Geometry check sheet. Reference: the model listing, model coordinates, mm. A direction names the side the tool comes from. Round coordinates to 2 decimals unless told otherwise and drop trailing zeros. Loops run counter-clockwise (first coordinate to the right, second up) from the corner with the lowest first, then second, coordinate; pieces in that order, holes last. Notation, with made-up numbers: (81, -18) - (124, -18) arc R16 ccw to (124, -14) - close; hole circle Ø2 at (-37, 59). An arc over 180 degrees is marked (long way). Answer as CSV lines item,"result". Start each with the question number.
1) Draft check along X on faces 3 (the cylindrical face through (98.013, 3.131, -136.616)), 4 (the flat face through (79, 0, -132)), 5 (the flat face through (160, 3, -128)). Enter one of: released by +X, released by -X, zero draft, split by the parting line, or undercut.
2) Depth check by flat-ended pin: P1, Ø3.5, axis at x = 118.12, z = -223.04, coming from the +Y side. Enter the tip coordinate at first touch or a pass-through.
3) Access from +Z, -Z, +X, -X, +Y, -Y to the whole of each face (thin tool, end or side, straight path). Record for faces 1 (the flat face through (71.65, 3, -10)), 2 (the flat face through (79, 3, -260)).
4) Cross-section at A-A on z = -45. Record the boundary of the cut face in (x, y), and give its area (4 significant figures).
5) Cross-section at C-C on y = 4.75. State how many separate pieces and enclosed holes the cut face has, and give its area (3 significant figures).
6) Cross-section at B-B on z = -193. Record the boundary of the cut face in (x, y).
7) Thickness scan on line 1 along X through (y, z) = (4.5, -170); line 2 along X through (y, z) = (4, -169.5); line 3 along Z through (x, y) = (84, 0.75). Record the ranges inside material, lowest first.
from build123d import *

# Parameters (mm, degrees)
SKETCH1_W           = 160
SKETCH1_H           = 260
SKETCH1_R           = 35
SKETCH1_R_2         = 25
SKETCH1_R_3         = 2.25
SKETCH1_R_4         = 1.175
SKETCH1_R_5         = 1.65
BOSS_EXTRUDE1_DEPTH = 6.35


with BuildPart() as part:
    # Sketch1 → Boss-Extrude1 (new body)
    with BuildSketch(Plane(origin=(0, 0, 0), x_dir=(1, 0, 0), z_dir=(0, 1, 0))):
        with Locations((80, 130)):
            Rectangle(SKETCH1_W, SKETCH1_H)
        with Locations(Location((87.5, 170, 0), (0, 0, 270))):
            Circle(SKETCH1_R, mode=Mode.SUBTRACT)
        with Locations(Location((87.5, 45, 0), (0, 0, 270))):
            Circle(SKETCH1_R_2, mode=Mode.SUBTRACT)
        with Locations(Location((148.75, 170, 0), (0, 0, 270))):
            Circle(SKETCH1_R_3, mode=Mode.SUBTRACT)
        with Locations(Location((118.125, 116.955944018, 0), (0, 0, 270))):
            Circle(SKETCH1_R_3, mode=Mode.SUBTRACT)
        with Locations(Location((56.875, 116.955944018, 0), (0, 0, 270))):
            Circle(SKETCH1_R_3, mode=Mode.SUBTRACT)
        with Locations(Location((26.25, 170, 0), (0, 0, 270))):
            Circle(SKETCH1_R_3, mode=Mode.SUBTRACT)
        with Locations(Location((56.875, 223.044055982, 0), (0, 0, 270))):
            Circle(SKETCH1_R_3, mode=Mode.SUBTRACT)
        with Locations(Location((118.125, 223.044055982, 0), (0, 0, 270))):
            Circle(SKETCH1_R_3, mode=Mode.SUBTRACT)
        with Locations(Location((5.475532842, 135.298909731, 0), (0, 0, 270))):
            Circle(SKETCH1_R_4, mode=Mode.SUBTRACT)
        with Locations(Location((9.516263037, 126.701090269, 0), (0, 0, 270))):
            Circle(SKETCH1_R_4, mode=Mode.SUBTRACT)
        with Locations(Location((10, 250, 0), (0, 0, 270))):
            Circle(SKETCH1_R_5, mode=Mode.SUBTRACT)
        with Locations(Location((30, 250, 0), (0, 0, 270))):
            Circle(SKETCH1_R_5, mode=Mode.SUBTRACT)
        with Locations(Location((50, 250, 0), (0, 0, 270))):
            Circle(SKETCH1_R_5, mode=Mode.SUBTRACT)
        with Locations(Location((70, 250, 0), (0, 0, 270))):
            Circle(SKETCH1_R_5, mode=Mode.SUBTRACT)
        with Locations(Location((90, 250, 0), (0, 0, 270))):
            Circle(SKETCH1_R_5, mode=Mode.SUBTRACT)
        with Locations(Location((110, 250, 0), (0, 0, 270))):
            Circle(SKETCH1_R_5, mode=Mode.SUBTRACT)
        with Locations(Location((130, 250, 0), (0, 0, 270))):
            Circle(SKETCH1_R_5, mode=Mode.SUBTRACT)
        with Locations(Location((150, 250, 0), (0, 0, 270))):
            Circle(SKETCH1_R_5, mode=Mode.SUBTRACT)
        with BuildLine():
            Line((8.35, 6.5), (8.35, 13.5))
            ThreePointArc((8.35, 13.5), (10, 15.15), (11.65, 13.5))
            Line((11.65, 13.5), (11.65, 6.5))
            ThreePointArc((11.65, 6.5), (10, 4.85), (8.35, 6.5))
        make_face(mode=Mode.SUBTRACT)
        with BuildLine():
            Line((31.65, 6.5), (31.65, 13.5))
            ThreePointArc((31.65, 13.5), (30, 15.15), (28.35, 13.5))
            Line((28.35, 13.5), (28.35, 6.5))
            ThreePointArc((28.35, 6.5), (30, 4.85), (31.65, 6.5))
        make_face(mode=Mode.SUBTRACT)
        with BuildLine():
            Line((51.65, 6.5), (51.65, 13.5))
            ThreePointArc((51.65, 13.5), (50, 15.15), (48.35, 13.5))
            Line((48.35, 13.5), (48.35, 6.5))
            ThreePointArc((48.35, 6.5), (50, 4.85), (51.65, 6.5))
        make_face(mode=Mode.SUBTRACT)
        with BuildLine():
            Line((71.65, 6.5), (71.65, 13.5))
            ThreePointArc((71.65, 13.5), (70, 15.15), (68.35, 13.5))
            Line((68.35, 13.5), (68.35, 6.5))
            ThreePointArc((68.35, 6.5), (70, 4.85), (71.65, 6.5))
        make_face(mode=Mode.SUBTRACT)
        with BuildLine():
            Line((91.65, 6.5), (91.65, 13.5))
            ThreePointArc((91.65, 13.5), (90, 15.15), (88.35, 13.5))
            Line((88.35, 13.5), (88.35, 6.5))
            ThreePointArc((88.35, 6.5), (90, 4.85), (91.65, 6.5))
        make_face(mode=Mode.SUBTRACT)
        with BuildLine():
            Line((111.65, 6.5), (111.65, 13.5))
            ThreePointArc((111.65, 13.5), (110, 15.15), (108.35, 13.5))
            Line((108.35, 13.5), (108.35, 6.5))
            ThreePointArc((108.35, 6.5), (110, 4.85), (111.65, 6.5))
        make_face(mode=Mode.SUBTRACT)
        with BuildLine():
            Line((131.65, 6.5), (131.65, 13.5))
            ThreePointArc((131.65, 13.5), (130, 15.15), (128.35, 13.5))
            Line((128.35, 13.5), (128.35, 6.5))
            ThreePointArc((128.35, 6.5), (130, 4.85), (131.65, 6.5))
        make_face(mode=Mode.SUBTRACT)
        with BuildLine():
            Line((151.65, 6.5), (151.65, 13.5))
            ThreePointArc((151.65, 13.5), (150, 15.15), (148.35, 13.5))
            Line((148.35, 13.5), (148.35, 6.5))
            ThreePointArc((148.35, 6.5), (150, 4.85), (151.65, 6.5))
        make_face(mode=Mode.SUBTRACT)
    extrude(amount=BOSS_EXTRUDE1_DEPTH)


solid = part.part
Answer block:
1,face 3,"undercut"
1,face 4,"zero draft"
1,face 5,"released by +X"
2,P1,"passes through"
3,face 1,"+Y, -Y"
3,face 2,"-Z, +X, -X, +Y, -Y"
4,outline,"(0, 0) - (62.5, 0) - (62.5, 6.35) - (0, 6.35) - close; (112.5, 0) - (160, 0) - (160, 6.35) - (112.5, 6.35) - close"
4,area,"698.5 mm^2"
5,separate pieces,"1"
5,enclosed holes,"26"
5,area,"35,400 mm^2"
6,outline,"(0, 0) - (61.12, 0) - (61.12, 6.35) - (0, 6.35) - close; (113.88, 0) - (160, 0) - (160, 6.35) - (113.88, 6.35) - close"
7,line 1,"x = 0 to 24, 28.5 to 52.5, 122.5 to 146.5, 151 to 160"
7,line 2,"x = 0 to 24.06, 28.44 to 52.5, 122.5 to 146.56, 150.94 to 160"
7,line 3,"z = -260 to -204.82, -135.18 to -69.75, -20.25 to 0"
